from build123d import *
from build123d.topology import SkipClean

# Parameters (mm, degrees)
CROQUIS1_R              = 6.5
SALIENTE_EXTRUIR1_DEPTH = 10
SALIENTE_EXTRUIR2_START = 4
CROQUIS2_R              = 16
SALIENTE_EXTRUIR2_DEPTH = 4
CROQUIS3_R              = 6.5
CORTAR_EXTRUIR1_DEPTH   = 4
SALIENTE_EXTRUIR3_DEPTH = 6
NERVIO1_REACH           = 84.68
CROQUIS5_WALL_W         = 215.909157244
CROQUIS5_WALL_H         = 10
NERVIO1_DRAFT_ANGLE     = -1
CHAFL_N3_SIZE           = 4
REDONDEO1_R             = 13
REDONDEO2_R             = 13
CROQUIS6_R              = 6.5
CORTAR_EXTRUIR2_DEPTH   = 6


with BuildPart() as part:
    # Croquis1 → Saliente-Extruir1 (new body)
    with BuildSketch(Plane.XY):
        with BuildLine():
            Line((-16, 0), (-16, -42))
            ThreePointArc((-16, -42), (-20.686291501, -53.313708499), (-32, -58))
            Line((-32, -58), (-38, -58))
            Line((-38, -58), (-38, -64))
            Line((-38, -64), (38, -64))
            Line((38, -64), (38, -58))
            Line((38, -58), (32, -58))
            ThreePointArc((32, -58), (20.686291501, -53.313708499), (16, -42))
            Line((16, -42), (16, 0))
            ThreePointArc((16, 0), (0, 16), (-16, 0))
        make_face()
        Circle(CROQUIS1_R, mode=Mode.SUBTRACT)
    extrude(amount=SALIENTE_EXTRUIR1_DEPTH)

    # Croquis2 → Saliente-Extruir2 (add)
    with SkipClean():  # the faces are left unmerged after this step: merging them gives an invalid solid
        with BuildSketch(Plane(origin=(0, 0, 0), x_dir=(-1, 0, 0), z_dir=(0, 0, -1)).offset(SALIENTE_EXTRUIR2_START)):
            Circle(CROQUIS2_R)
        extrude(amount=-SALIENTE_EXTRUIR2_DEPTH)

    # Croquis3 → Cortar-Extruir1 (cut)
    with SkipClean():  # the faces are left unmerged after this step: merging them gives an invalid solid
        with BuildSketch(Plane(origin=(0, 0, -4), x_dir=(-1, 0, 0), z_dir=(0, 0, -1))):
            Circle(CROQUIS3_R)
        extrude(amount=-CORTAR_EXTRUIR1_DEPTH, mode=Mode.SUBTRACT)

    # Croquis4 → Saliente-Extruir3 (add)
    with SkipClean():  # the faces are left unmerged after this step: merging them gives an invalid solid
        with BuildSketch(Plane.XZ.offset(64)):
            Polygon((38, 0), (38, 36), (-38, 36), (-38, -4), (38, -4), align=None)
        extrude(amount=-SALIENTE_EXTRUIR3_DEPTH)

    # Croquis5 wall → Nervio1 (add, up to next)
    with BuildSketch(Plane(origin=(0, -37.5, 23), x_dir=(0, 0.84450857845, -0.535542025358), z_dir=(0, 0.535542025358, 0.84450857845)), mode=Mode.PRIVATE) as nervio1_sk1:
        Rectangle(CROQUIS5_WALL_W, CROQUIS5_WALL_H)
    nervio1_tool1 = extrude(nervio1_sk1.sketch, amount=-NERVIO1_REACH, mode=Mode.PRIVATE) - part.part
    add(nervio1_tool1.solids().sort_by_distance((0, -37.5, 23))[0])

    # Nervio1 draft
    nervio1_draft_faces = [part.faces().sort_by_distance(p)[0] for p in [
        (-5, -37.767771013, 22.577745711),
        (5, -37.767771013, 22.577745711),
    ]]
    draft(nervio1_draft_faces, Plane(origin=(0, -37.5, 23), x_dir=(0, 0.84450857845, -0.535542025358), z_dir=(0, 0.535542025358, 0.84450857845)), NERVIO1_DRAFT_ANGLE)

    # Chaflán3
    chafl_n3_edges = [part.edges().sort_by_distance(p)[0] for p in [
        (0, -58, -4),
    ]]
    chamfer(chafl_n3_edges, length=CHAFL_N3_SIZE - 0.0001)  # a hair under: the kernel refuses the full size

    # Redondeo1
    redondeo1_edges = [part.edges().sort_by_distance(p)[0] for p in [
        (-38, -61, 36),
    ]]
    fillet(redondeo1_edges, radius=REDONDEO1_R)

    # Redondeo2
    redondeo2_edges = [part.edges().sort_by_distance(p)[0] for p in [
        (38, -61, 36),
    ]]
    fillet(redondeo2_edges, radius=REDONDEO2_R)

    # Croquis6 → Cortar-Extruir2 (cut)
    with BuildSketch(Plane(origin=(0, -58, 0), x_dir=(1, 0, 0), z_dir=(0, 1, 0))):
        with Locations(Location((-25, -23, 0), (0, 0, 270))):
            Circle(CROQUIS6_R)
        with Locations(Location((25, -23, 0), (0, 0, 270))):
            Circle(CROQUIS6_R)
    extrude(amount=-CORTAR_EXTRUIR2_DEPTH, mode=Mode.SUBTRACT)


solid = part.part
Could you check a few things on this model? Use its own coordinates, in mm. Give positions to 0.01 mm unless a question says otherwise; leave off trailing zeros. Order: outer loops, then holes, each group sorted by start corner. A loop starts at its lowest first (then second) coordinate and runs counter-clockwise, first axis right, second up. Notation, with made-up numbers: (-12, -22) -> (47, -22) arc R16 cw to (47, -8) -> close; hole circle Ø6 at (74, 52). An arc over 180 degrees is marked (long way). Answer in a Markdown table with one row per item. Add a question column.
Item 1: Imagine slicing it at C-C (z = 25). List the corners of the cut face in (x, y) for me.
Item 2: Imagine slicing it at A-A (z = 7). List the corners of the cut face in (x, y) for me.
Item 3: We'd pull the mould along X, two halves only. Please class faces 1 (the cylindrical face through (34.091, -60.958, 32.293)), 2 (the cylindrical face through (-20.563, -53.189, 4.93)), 3 (the flat face through (-1, -60, -2)), 4 (the cylindrical face through (25.286, -60.958, 16.506)): pulls with the +X half, pulls with the -X half, needs draft (parallel to the pull), parting line crosses it, or undercut.
Item 4: Please list where these lines run through material, in increasing order: probe 1 along X at (y, z) = (-61, 23); probe 2 along Y at (x, z) = (0, 4.5); probe 3 along Y at (x, z) = (-28, 31).
Item 5: I'm going to push flat-ended pins straight in: P1, Ø8, axis at y = 5.5, z = 12.5, coming from the +X side; P2, Ø2, axis at x = 10.5, y = -24, coming from the -Z side; P3, Ø17, axis at x = 25, z = 23, coming from the +Y side; P4, Ø15, axis at x = 0, y = 0, coming from the -Z side. Where does each tip first touch, or does it pass through?
Item 6: Imagine slicing it at D-D (y = -28.5). List the corners of the cut face in (x, z) for me.
Result:
| question | item | result |
|---|---|---|
| 1 | outline | (-37.85, -64) -> (-31.18, -64) -> (-31.18, -58) -> (-37.85, -58) -> close; (-18.82, -64) -> (18.82, -64) -> (18.82, -58) -> (4.84, -58) -> (5, -40.65) -> (-5, -40.65) -> (-4.84, -58) -> (-18.82, -58) -> close; (31.18, -64) -> (37.85, -64) -> (37.85, -58) -> (31.18, -58) -> close |
| 2 | outline | (-38, -64) -> (38, -64) -> (38, -58) -> (32, -58) arc R16 cw to (16, -42) -> (16, 0) arc R16 ccw to (-16, 0) -> (-16, -42) arc R16 cw to (-32, -58) -> (-38, -58) -> close; hole circle Ø13 at (0, 0) |
| 3 | face 1 | pulls with the +X half |
| 3 | face 2 | pulls with the -X half |
| 3 | face 3 | needs draft |
| 3 | face 4 | undercut |
| 4 | probe 1 | -38 to -31.5, -18.5 to 18.5, 31.5 to 38 |
| 4 | probe 2 | -64 to -6.5, 6.5 to 16 |
| 4 | probe 3 | -64 to -58 |
| 5 | P1 | x = 15.82 |
| 5 | P2 | z = 0 |
| 5 | P3 | y = -58 |
| 5 | P4 | z = -4 |
| 6 | outline | (-16, 0) -> (16, 0) -> (16, 10) -> (4.89, 10) -> (5, 17.29) -> (-5, 17.29) -> (-4.89, 10) -> (-16, 10) -> close |
